Design review of the part built by this model. Coordinates are the model's own, in mm. A direction names the side the tool comes from. Give positions to 0.01 mm unless a question says otherwise; leave off trailing zeros. Order: outer loops, then holes, each group sorted by start corner. A loop starts at its lowest first (then second) coordinate and runs counter-clockwise, first axis right, second up. Notation, with made-up numbers: M 4.5,-25 L 9.5,-25 A18 ccw 9.5,-10 Z; hole C -3,-14 d9. An arc over 180 degrees is marked long. Put each result on its own line as item: value. Start each with the question number.
Solid Edge part; units mm, degrees
sketch "Sketch1" plane through (0, 0, 0) normal (0, 0, 1) x (1, 0, 0)
  line L0 (49.1, 16) -> (49.1, 21)
  line L1 (49.1, 21) -> (19.1, 21)
  line L2 (19.1, 21) -> (19.1, 16)
  line L3 (19.1, 16) -> (49.1, 16)
  line L4 (5, -39.5) -> (7, -39.5)
  line L5 (7, -39.5) -> (7, -14.5)
  line L6 (7, -14.5) -> (5, -14.5)
  line L7 (5, -14.5) -> (5, -39.5)
  line L8 (51.1, 41.5) -> (-51.1, 41.5)
  line L9 (-51.1, 41.5) -> (-51.1, -41.5)
  line L10 (-51.1, -41.5) -> (51.1, -41.5)
  line L11 (51.1, -41.5) -> (51.1, 41.5)
  line L12 (-19.1, 16) -> (-49.1, 16)
  line L13 (-49.1, 16) -> (-49.1, 21)
  line L14 (-49.1, 21) -> (-19.1, 21)
  line L15 (-19.1, 21) -> (-19.1, 16)
  line L16 (-5, -39.5) -> (-7, -39.5)
  line L17 (-7, -39.5) -> (-7, -14.5)
  line L18 (-7, -14.5) -> (-5, -14.5)
  line L19 (-5, -14.5) -> (-5, -39.5)
extrude "Protrusion1" add sketch "Sketch1" along normal blind 2
sketch "Sketch2" plane through (0, 0, 2) normal (0, 0, 1) x (1, 0, 0)
  circle A0 centre (-42.5, -25) radius 1.2
  circle A1 centre (-42.5, -25) radius 2.4
  circle A2 centre (42.5, 25) radius 2.4
  circle A3 centre (42.5, 25) radius 1.2
extrude "ProtrusiónExtruida_2" add sketch "Sketch2" along normal blind 6.2
sketch "Sketch3" plane through (0, 0, 2) normal (0, 0, 1) x (1, 0, 0)
  line L0 (51.1, 41.5) -> (-51.1, 41.5)
  line L1 (-51.1, 41.5) -> (-51.1, 5)
  line L2 (-51.1, 5) -> (-53.5, 5)
  line L3 (-53.5, 5) -> (-53.5, 43.85)
  line L4 (-53.5, 43.85) -> (53.5, 43.85)
  line L5 (53.5, 43.85) -> (53.5, 5)
  line L6 (53.5, 5) -> (51.1, 5)
  line L7 (51.1, 5) -> (51.1, 41.5)
  line L8 (-53.5, -43.85) -> (53.5, -43.85)
  line L9 (53.5, -43.85) -> (53.5, -5)
  line L10 (53.5, -5) -> (51.1, -5)
  line L11 (51.1, -5) -> (51.1, -41.5)
  line L12 (51.1, -41.5) -> (-51.1, -41.5)
  line L13 (-51.1, -41.5) -> (-51.1, -5)
  line L14 (-51.1, -5) -> (-53.5, -5)
  line L15 (-53.5, -5) -> (-53.5, -43.85)
extrude "ProtrusiónExtruida_7" add sketch "Sketch3" against normal blind 2 and the other way blind 6.9
sketch "Sketch4" plane through (0, -24.425, 8.9) normal (0, 0, 1) x (1, 0, 0)
  line L0 (-51.1, 29.425) -> (-51.1, 65.925)
  line L1 (-51.1, 65.925) -> (51.1, 65.925)
  line L2 (51.1, 65.925) -> (51.1, 29.425)
  line L3 (51.1, 29.425) -> (52.1, 29.425)
  line L4 (52.1, 29.425) -> (52.1, 66.925)
  line L5 (52.1, 66.925) -> (-52.1, 66.925)
  line L6 (-52.1, 66.925) -> (-52.1, 29.423)
  line L7 (-52.1, 29.423) -> (-51.1, 29.425)
  line L8 (52.1, -18.075) -> (-52.1, -18.075)
  line L9 (-52.1, -18.075) -> (-52.1, 19.427)
  line L10 (-52.1, 19.427) -> (-51.1, 19.425)
  line L11 (-51.1, 19.425) -> (-51.1, -17.075)
  line L12 (-51.1, -17.075) -> (51.1, -17.075)
  line L13 (51.1, -17.075) -> (51.1, 19.425)
  line L14 (51.1, 19.425) -> (52.1, 19.425)
  line L15 (52.1, 19.425) -> (52.1, -18.075)
extrude "ProtrusiónExtruida_8" add sketch "Sketch4" along normal blind 1
sketch "Sketch5" plane through (0, 0, 2) normal (0, 0, 1) x (1, 0, 0)
  line L0 (-49.65, 5.6) -> (-49.65, -5.6)
  line L1 (-49.65, -5.6) -> (-51.1, -5.6)
  line L2 (-51.1, -5.6) -> (-51.1, 5.6)
  line L3 (-51.1, 5.6) -> (-49.65, 5.6)
  line L4 (49.65, 5.6) -> (49.65, -5.6)
  line L5 (49.65, -5.6) -> (51.1, -5.6)
  line L6 (51.1, -5.6) -> (51.1, 5.6)
  line L7 (51.1, 5.6) -> (49.65, 5.6)
extrude "ProtrusiónExtruida_9" add sketch "Sketch5" along normal blind 7
sketch "Sketch6" plane through (50.375, 0, 9) normal (0, 0, 1) x (0, 1, 0)
  line L0 (2.3332, 0.725) -> (-2.5, 0.725)
  line L1 (-2.5, 0.725) -> (-2.5, -0.725)
  line L2 (-2.5, -0.725) -> (2.3332, -0.725)
  line L3 (2.3332, -0.725) -> (2.3332, 0.725)
  line L4 (-2.5, 101.475) -> (2.3332, 101.475)
  line L5 (2.3332, 101.475) -> (2.3332, 100.025)
  line L6 (2.3332, 100.025) -> (-2.5, 100.025)
  line L7 (-2.5, 100.025) -> (-2.5, 101.475)
extrude "Protrusion2" add sketch "Sketch6" along normal blind 3
sketch "Sketch7" plane through (-50.375, -2.5, 14.95) normal (0, -1, 0) x (0, 0, 1)
  line L0 (1.05, -0.725) -> (-2.95, -0.725)
  line L1 (-2.95, -0.725) -> (-2.95, 0.725)
  line L2 (-2.95, 0.725) -> (-2.95, 2.775)
  line L3 (-2.95, 2.775) -> (-2.0269, 2.775)
  line L4 (-2.0269, 2.775) -> (1.05, 0.775)
  line L5 (1.05, 0.775) -> (1.05, -0.725)
extrude "Protrusion3" add sketch "Sketch7" against normal up to surface (4.8332 mm away)
sketch "Sketch8" plane through (-50.375, -2.5, 14.95) normal (0, -1, 0) x (0, 0, 1)
  line L0 (-2.95, -100.025) -> (-2.95, -101.475)
  line L1 (-2.95, -101.475) -> (-2.95, -103.525)
  line L2 (-2.95, -103.525) -> (-2.0269, -103.525)
  line L3 (-2.0269, -103.525) -> (1.05, -101.525)
  line L4 (1.05, -101.525) -> (1.05, -100.025)
  line L5 (1.05, -100.025) -> (-2.95, -100.025)
extrude "Protrusion4" add sketch "Sketch8" against normal up to surface (4.8332 mm away)
sketch "Sketch9" plane through (51.1, 0, 6) normal (1, 0, 0) x (0, 1, 0)
  line L0 (-17.7511, -6) -> (17.7489, -6)
  line L1 (17.7489, -6) -> (17.7489, -4.918)
  line L2 (17.7489, -4.918) -> (-17.7511, -4.918)
  line L3 (-17.7511, -4.918) -> (-17.7511, -6)
extrude "Cutout1" cut sketch "Sketch9" against normal up to surface (107 mm away) from surface at 2.4
sketch "Sketch10" plane through (0, -43.85, 4.45) normal (0, -1, 0) x (1, 0, 0)
  line L0 (7, -3.45) -> (-7, -3.45)
  line L1 (-7, -3.45) -> (-7, -4.45)
  line L2 (-7, -4.45) -> (7, -4.45)
  line L3 (7, -4.45) -> (7, -3.45)
extrude "Cutout2" cut sketch "Sketch10" against normal up to surface (4.35 mm away)
1. Consider section B-B on y = -25. Give the boundary of the cut face in (x, z), then the cut area to 3 significant figures.
2. Consider section D-D on y = 25. Give the boundary of the cut face in (x, z).
3. Consider section A-A on z = 6.5. Give the boundary of the cut face in (x, y), then the cut area to 3 significant figures.
4. To check wall thickness, follow probe 1 along Y at (x, z) = (-42.5, 6); probe 2 along Y at (x, z) = (13, 7.5); probe 3 along Y at (x, z) = (42.5, 4.75). State the ranges of each line that lie inside material, in increasing order.
5. Insertion check: pin 1 (1 mm diameter, centred on x = 28.5, y = 4, fed in from +Z); pin 2 (3 mm diameter, centred on y = 0.5, z = 4, fed in from -X); pin 3 (1.8 mm diameter, centred on x = -52, z = 12.5, fed in from -Y). Each pin has a flat end and moves straight along its axis. Give the tip position at first contact, or say it passes through.
6. Consider section C-C on x = 42.5. Give the boundary of the cut face in (y, z).
7. Machinability: for faces 1 (the flat face through (41, 25, 8.2)), 2 (the flat face through (0, -28, 0)), 3 (the flat face through (-52, -5, 5)), which of the approach directions +Z, -Z, +X, -X, +Y, -Y give a long, thin tool a straight path to every point of the face, cutting with its end or side? Answer none if there is none.
8. The part is to be moulded in two halves that separate along Y. For faces 4 (the flat face through (52, 5, 6)), 5 (the flat face through (53.5, -25, 5)), say which applies: +Y half, -Y half, draft (parallel to the pull), parting line (faces both ways), or undercut.
Returned:
1. outline: M -53.5,0 L -7,0 L -7,2 L -40.1,2 L -40.1,8.2 L -41.3,8.2 L -41.3,2 L -43.7,2 L -43.7,8.2 L -44.9,8.2 L -44.9,2 L -51.1,2 L -51.1,9.9 L -52.1,9.9 L -52.1,8.9 L -53.5,8.9 Z; M -5,0 L 5,0 L 5,2 L -5,2 Z; M 7,0 L 53.5,0 L 53.5,8.9 L 52.1,8.9 L 52.1,9.9 L 51.1,9.9 L 51.1,2 L 7,2 Z
1. area: 256 mm2
2. outline: M -53.5,0 L 53.5,0 L 53.5,8.9 L 52.1,8.9 L 52.1,9.9 L 51.1,9.9 L 51.1,2 L 44.9,2 L 44.9,8.2 L 43.7,8.2 L 43.7,2 L 41.3,2 L 41.3,8.2 L 40.1,8.2 L 40.1,2 L -51.1,2 L -51.1,9.9 L -52.1,9.9 L -52.1,8.9 L -53.5,8.9 Z
3. outline: M -53.5,-43.85 L 53.5,-43.85 L 53.5,-5 L 51.1,-5 L 51.1,5 L 53.5,5 L 53.5,43.85 L -53.5,43.85 L -53.5,5 L -51.1,5 L -51.1,-5 L -53.5,-5 Z; C -42.5,-25 d4.8; C 42.5,25 d4.8; hole M -51.1,-41.5 L 51.1,-41.5 L 51.1,-5.6 L 49.65,-5.6 L 49.65,5.6 L 51.1,5.6 L 51.1,41.5 L -51.1,41.5 L -51.1,5.6 L -49.65,5.6 L -49.65,-5.6 L -51.1,-5.6 Z; hole C -42.5,-25 d2.4; hole C 42.5,25 d2.4
3. area: 913 mm2
4. probe 1: y = -43.85 to -41.5, -27.4 to -26.2, -23.8 to -22.6, 41.5 to 43.85
4. probe 2: y = -43.85 to -41.5, 41.5 to 43.85
4. probe 3: y = -43.85 to -41.5, 22.6 to 23.8, 26.2 to 27.4, 41.5 to 43.85
5. pin 1: stops at z = 2
5. pin 2: stops at x = -51.1
5. pin 3: stops at y = -2.5
6. outline: M -43.85,0 L -17.75,0 L -17.75,1.08 L 16,1.08 L 16,2 L -41.5,2 L -41.5,9.9 L -42.5,9.9 L -42.5,8.9 L -43.85,8.9 Z; M 21,0 L 43.85,0 L 43.85,8.9 L 42.5,8.9 L 42.5,9.9 L 41.5,9.9 L 41.5,2 L 27.4,2 L 27.4,8.2 L 26.2,8.2 L 26.2,2 L 23.8,2 L 23.8,8.2 L 22.6,8.2 L 22.6,2 L 21,2 Z
7. face 1: +Z
7. face 2: -Z, +X, -X, +Y, -Y
7. face 3: +Z, -Z, -X
8. face 4: undercut
8. face 5: draft
